Input: part model. Units: mm. Frame: model coordinates. A direction names the side the tool comes from. Round coordinates to 2 decimals unless told otherwise and drop trailing zeros. Order: outer loops, then holes, each group sorted by start corner. A loop starts at its lowest first (then second) coordinate and runs counter-clockwise, first axis right, second up. Notation, with made-up numbers: (-34, 78.25) -> (10, 78.25) arc R12 ccw to (10, 97.25) -> close; hole circle Ø5 at (-22, 68.25). An arc over 180 degrees is marked (long way). Use a Markdown table: item, result.
from build123d import *

# Parameters (mm, degrees)
SKETCH_1_R          = 40
EXTRUDE_1_DEPTH     = 200
SKETCH_2_R          = 20
CUT_EXTRUDE_1_DEPTH = 150
CHAMFER_1_SIZE      = 2
FILLET_1_R          = 1
FILLET_2_R          = 1


with BuildPart() as part:
    # Эскиз1 → Бобышка-Вытянуть1 (new body)
    with BuildSketch(Plane(origin=(0, 0, 0), x_dir=(1, 0, 0), z_dir=(0, 1, 0))):
        with Locations(Location((0, 0, 0), (0, 0, 270))):
            Circle(SKETCH_1_R)
    extrude(amount=EXTRUDE_1_DEPTH)

    # Эскиз2 → Вырез-Вытянуть1 (cut)
    with BuildSketch(Plane(origin=(0, 200, 0), x_dir=(1, 0, 0), z_dir=(0, 1, 0))):
        with Locations(Location((0, 0, 0), (0, 0, 270))):
            Circle(SKETCH_2_R)
    extrude(amount=-CUT_EXTRUDE_1_DEPTH, mode=Mode.SUBTRACT)

    # Фаска1
    chamfer_1_edges = [part.edges().sort_by_distance(p)[0] for p in [
        (0, 200, -20),
    ]]
    chamfer(chamfer_1_edges, length=CHAMFER_1_SIZE)

    # Скругление1
    fillet_1_edges = [part.edges().sort_by_distance(p)[0] for p in [
        (0, 0, -40),
    ]]
    fillet(fillet_1_edges, radius=FILLET_1_R)

    # Скругление2
    fillet_2_edges = [part.edges().sort_by_distance(p)[0] for p in [
        (0, 200, -40),
    ]]
    fillet(fillet_2_edges, radius=FILLET_2_R)


solid = part.part
1) Set-up query: faces 4 (the face through (-17, 200, 17)), 5 (the face through (0, 50, 0)). Return all of +Z, -Z, +X, -X, +Y, -Y with unobstructed straight access to the full face (end or side cutting, diameter ignored); none if empty.
Answer key:
| item | result |
|---|---|
| face 4 | +Z, -Z, +X, -X, +Y |
| face 5 | +Y |
2) Cut plane A-A on z = 0. Return loops of the section in (x, y).
Answer key:
| item | result |
|---|---|
| outline | (-40, 1) arc R1 ccw to (-39, 0) -> (39, 0) arc R1 ccw to (40, 1) -> (40, 199) arc R1 ccw to (39, 200) -> (22, 200) -> (20, 198) -> (20, 50) -> (-20, 50) -> (-20, 198) -> (-22, 200) -> (-39, 200) arc R1 ccw to (-40, 199) -> close |
3) Cut plane D-D on y = 25. Return loops of the section in (x, z).
Answer key:
| item | result |
|---|---|
| outline | circle Ø80 at (0, 0) |
4) Draft query along Z for faces 1 (the face through (-19.524, 125.036, -4.336)), 2 (the face through (-39.05, 98.61, -8.67)), 3 (the face through (1, 0, -1)). Return one class per face: released by +Z, released by -Z, zero draft, split by the parting line, or undercut.
Answer key:
| item | result |
|---|---|
| face 1 | undercut |
| face 2 | split by the parting line |
| face 3 | zero draft |
5) Cut plane B-B on x = 0. Return loops of the section in (y, z), and give its area (4 significant figures).
Answer key:
| item | result |
|---|---|
| outline | (0, -39) arc R1 ccw to (1, -40) -> (199, -40) arc R1 ccw to (200, -39) -> (200, -22) -> (198, -20) -> (50, -20) -> (50, 20) -> (198, 20) -> (200, 22) -> (200, 39) arc R1 ccw to (199, 40) -> (1, 40) arc R1 ccw to (0, 39) -> close |
| area | 10,000 mm^2 |
6) Cut plane C-C on y = 52. Return loops of the section in (x, z), and give its area (3 significant figures).
Answer key:
| item | result |
|---|---|
| outline | circle Ø80 at (0, 0); hole circle Ø40 at (0, 0) |
| area | 3,770 mm^2 |
7) Contact query for flat-ended pins moving along their axis: P1, Ø1.5, axis at y = 112.5, z = 17, coming from the +X side; P2, Ø5, axis at y = 90, z = -23.5, coming from the -X side; P3, Ø5, axis at x = 13, z = -13.5, coming from the -Y side; P4, Ø1, axis at x = -21, y = 154, coming from the -Z side. Output: stop coordinate, or through.
Answer key:
| item | result |
|---|---|
| P1 | stops at x = 36.55 |
| P2 | stops at x = -34.04 |
| P3 | stops at y = 0 |
| P4 | stops at z = -34.35 |
8) Ray query, probe 1 along X at (y, z) = (113, 0); probe 2 along Z at (x, y) = (-0.5, 72.5); probe 3 along Y at (x, z) = (4, 10.5). Return the intervals inside material, ascending.
Answer key:
| item | result |
|---|---|
| probe 1 | x = -40 to -20, 20 to 40 |
| probe 2 | z = -40 to -19.99, 19.99 to 40 |
| probe 3 | y = 0 to 50 |
